Verification items for the finished model (mm, model axes). Face numbers are marked on the shaded views. A direction names the side the tool comes from. Coordinates: 2 decimals unless noted, no trailing zeros. Order: outer loops, then holes, each group sorted by start corner. A loop starts at its lowest first (then second) coordinate and runs counter-clockwise, first axis right, second up. Notation, with made-up numbers: (88.25, -3.5) -> (147.25, -3.5) arc R17 cw to (147.25, 29.5) -> close; hole circle Ø6 at (32, -34). An arc over 180 degrees is marked (long way). Write each question's results on one line, items separated by ' | '. Start each with the question number.
(1) Draft check along X on the marked faces 5, 6, 7 and 8. Enter one of: +X half, -X half, draft (parallel to the pull), parting line (faces both ways), or undercut.
(2) Thickness scan on probe 1 along X at (y, z) = (-0.25, 0.3); probe 2 along Y at (x, z) = (-7, 0.25); probe 3 along Z at (x, y) = (-4.75, 1.75). Record the ranges inside material, lowest first. Write a range as [from, to].
(3) Cross-section at C-C on x = 0. Enter the section's corners in (y, z).
(4) Go/stop test with flat-tipped pins: pin 1 (1.6 mm diameter, centred on x = 0.5, z = 2.5, fed in from +Y); pin 2 (0.8 mm diameter, centred on x = 5.5, z = 0.5, fed in from +Y); pin 3 (1 mm diameter, centred on y = -4, z = 2.5, fed in from -X); pin 4 (0.5 mm diameter, centred on x = 6.5, z = 0.5, fed in from -Y). Record where each tip stops, or that it passes through.
(5) Cross-section at A-A on y = 0. Enter the section's corners in (x, z).
(6) Set-up check for the marked faces 1, 2, 3 and 4: record each of +Z, -Z, +X, -X, +Y, -Y from which the full face is reachable in a straight line by a thin tool's end or side.
(7) Cross-section at B-B on z = 0.2. Enter the section's corners in (x, y), and give its area (3 significant figures).
(8) Cross-section at D-D on y = 3. Enter the section's corners in (x, z).
Autodesk Inventor part; units mm, degrees
ref_plane "YZ Plane" through (0, 0, 0) normal (1, 0, 0) x (0, 1, 0)
ref_plane "XZ Plane" through (0, 0, 0) normal (0, 1, 0) x (-1, 0, 0)
ref_plane "XY Plane" through (0, 0, 0) normal (0, 0, 1) x (1, 0, 0)
sketch "Náčrt1" plane through (0, 0, 0) normal (0, 0, 1) x (1, 0, 0)
  line L0 (-5, 5.75) -> (5, 5.75)
  line L1 (5, -5.75) -> (-5, -5.75)
  line L2 (-5, 5.75) -> (5, -5.75) construction
  line L3 (5, 5.75) -> (-5, -5.75) construction
  line L4 (-5, 2.5) -> (-7.5, 2.5)
  arc A0 (-7.5, 2.5) -> (-7.5, -2.5) centre (-7.5, 0) ccw
  line L5 (-7.5, -2.5) -> (-5, -2.5)
  line L6 (5, 2.5) -> (7.5, 2.5)
  arc A1 (7.5, -2.5) -> (7.5, 2.5) centre (7.5, 0) ccw
  line L7 (7.5, -2.5) -> (5, -2.5)
  line L8 (-5, -5.75) -> (-5, -2.5)
  line L9 (-5, 2.5) -> (-5, 5.75)
  line L10 (5, 5.75) -> (5, 2.5)
  line L11 (5, -2.5) -> (5, -5.75)
  line L12 (-7.5, 0) -> (-7, 0) construction
  line L13 (-7.5, -1) -> (-7, -1)
  line L14 (-7, 1) -> (-7.5, 1)
  arc A2 (-7.5, 1) -> (-7.5, -1) centre (-7.5, 0) ccw
  arc A3 (-7, -1) -> (-7, 1) centre (-7, 0) ccw
  line L15 (7.5, 0) -> (7, 0) construction
  line L16 (7.5, 1) -> (7, 1)
  line L17 (7, -1) -> (7.5, -1)
  arc A4 (7.5, -1) -> (7.5, 1) centre (7.5, 0) ccw
  arc A5 (7, 1) -> (7, -1) centre (7, 0) ccw
  point P0 (0, 0)
  point P1 (-7.25, 0)
  point P2 (7.25, 0)
  point P3 (10, 0)
  point P4 (-10, 0)
  point P5 (-6, 0)
  point P6 (-8.5, 0)
  dimension "d0" = 11.5
  dimension "d1" = 10
  dimension "d2" = 5
  dimension "d3" = 2
  dimension "d4" = 20
  dimension "d5" = 2.5
extrude "Vysunutí1" add sketch "Náčrt1" along normal blind 1
sketch "Náčrt2" plane through (0, 0, 1) normal (0, 0, 1) x (1, 0, 0)
  line L0 (-2.5, 0) -> (2.5, 0) construction
  line L1 (2.5, -3.25) -> (-2.5, -3.25)
  arc A0 (-2.5, 3.25) -> (-2.5, -3.25) centre (-2.5, 0) ccw
  arc A1 (2.5, -3.25) -> (2.5, 3.25) centre (2.5, 0) ccw
  arc A2 (1, 3.25) -> (-1, 3.25) centre (0, 3.25) ccw
  line L2 (-2.5, 3.25) -> (-1, 3.25)
  line L3 (1, 3.25) -> (2.5, 3.25)
  point P0 (0, 0)
  point P1 (5.75, 0)
  point P2 (-5.75, 0)
  dimension "d8" = 6.5
  dimension "d9" = 11.5
  dimension "d10" = 1
extrude "Vysunutí2" add sketch "Náčrt2" along normal blind 1
sketch "Náčrt3" plane through (0, 0, 2) normal (0, 0, 1) x (1, 0, 0)
  arc A0 (-2.5, 3.25) -> (-2.5, -3.25) centre (-2.5, 0) ccw
  line L0 (-1, 3.25) -> (-2.5, 3.25)
  line L1 (2.5, 3.25) -> (1, 3.25)
  arc A1 (2.5, -3.25) -> (2.5, 3.25) centre (2.5, 0) ccw
  line L2 (-2.5, -3.25) -> (2.5, -3.25)
  line L3 (-1, 3.25) -> (1, 3.25)
  line L4 (2.5, 2.5) -> (1, 2.5)
  line L5 (1, 2.5) -> (-1, 2.5)
  line L6 (-1, 2.5) -> (-2.5, 2.5)
  arc A2 (-2.5, 2.5) -> (-2.5, -2.5) centre (-2.5, 0) ccw
  line L7 (-2.5, -2.5) -> (2.5, -2.5)
  arc A3 (2.5, -2.5) -> (2.5, 2.5) centre (2.5, 0) ccw
  point P0 (0, 0)
  dimension "d13" = 0.75
extrude "Vysunutí3" add sketch "Náčrt3" along normal blind 1.5 contours A3 L7 A2 L6 L5 L4
properties part number "TF-LC02 (Laser senzor)"
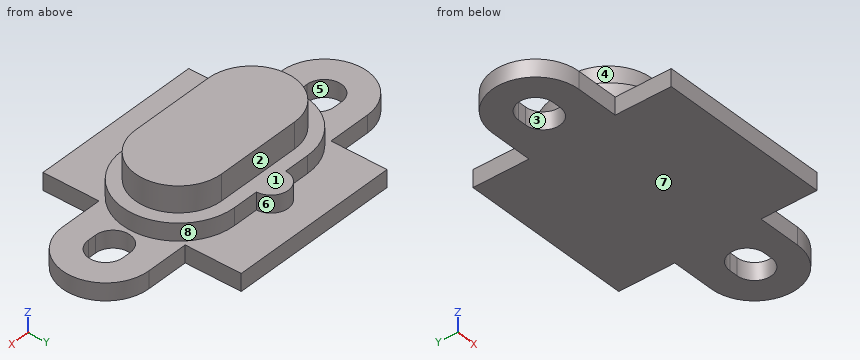
Results are:
1) face 5: undercut | face 6: parting line | face 7: draft | face 8: +X half
2) probe 1: x = [-9.99, -8.47], [-6.03, 6.03], [8.47, 9.99] | probe 2: y = [-2.5, -1], [1, 2.5] | probe 3: z = [0, 2]
3) outline: (-5.75, 0) -> (5.75, 0) -> (5.75, 1) -> (4.25, 1) -> (4.25, 2) -> (2.5, 2) -> (2.5, 3.5) -> (-2.5, 3.5) -> (-2.5, 2) -> (-3.25, 2) -> (-3.25, 1) -> (-5.75, 1) -> close
4) pin 1: stops at y = 4.25 | pin 2: stops at y = 2.5 | pin 3: passes through | pin 4: stops at y = -2.5
5) outline: (-10, 0) -> (-8.5, 0) -> (-8.5, 1) -> (-10, 1) -> close; (-6, 0) -> (6, 0) -> (6, 1) -> (5.75, 1) -> (5.75, 2) -> (5, 2) -> (5, 3.5) -> (-5, 3.5) -> (-5, 2) -> (-5.75, 2) -> (-5.75, 1) -> (-6, 1) -> close; (8.5, 0) -> (10, 0) -> (10, 1) -> (8.5, 1) -> close
6) face 1: +Z | face 2: +Z, +X, -X, +Y | face 3: +Z, -Z | face 4: +Z, -X
7) outline: (-7.5, -2.5) -> (-5, -2.5) -> (-5, -5.75) -> (5, -5.75) -> (5, -2.5) -> (7.5, -2.5) arc R2.5 ccw to (7.5, 2.5) -> (5, 2.5) -> (5, 5.75) -> (-5, 5.75) -> (-5, 2.5) -> (-7.5, 2.5) arc R2.5 ccw to start; hole (-7.5, -1) -> (-7, -1) arc R1 ccw to (-7, 1) -> (-7.5, 1) arc R1 ccw to start; hole (7, -1) -> (7.5, -1) arc R1 ccw to (7.5, 1) -> (7, 1) arc R1 ccw to start | area: 151 mm2
8) outline: (-5, 0) -> (5, 0) -> (5, 1) -> (3.75, 1) -> (3.75, 2) -> (-3.75, 2) -> (-3.75, 1) -> (-5, 1) -> close
